from build123d import *

# Parameters (mm, degrees)
F1_DEPTH = 45
F2_W     = 30
F2_H     = 13
F3_DEPTH = 3
F4_W     = 2.1
F4_H     = 6
F5_DEPTH = 11
F7_D     = 2.83
F7_DEPTH = 2
F7_TIP   = 0.8502177759
F8_W     = 2
F8_H     = 45
F9_DEPTH = 1.5
F10_R    = 0.5


with BuildPart() as f1:
    # F0 (on Front) → F1 (new body)
    with BuildSketch(Plane.XZ):
        Polygon((0, 16), (0, 0), (20, 0), (20, 1.5), (3, 1.5), (1.5, 16), align=None)
    extrude(amount=F1_DEPTH)

    # F2 (on face) → F3 (join)
    with BuildSketch(Plane(origin=(0, 0, 0), x_dir=(0, -1, 0), z_dir=(-1, 0, 0))):
        with Locations((22.5, 6.5)):
            Rectangle(F2_W, F2_H)
    extrude(amount=F3_DEPTH)

    # F4 (on face) → F5 (cut)
    with BuildSketch(Plane(origin=(0, 0, 0), x_dir=(1, 0, 0), z_dir=(0, 0, -1))):
        with Locations((-1.05, 33.5)):
            Rectangle(F4_W, F4_H)
        with Locations((-1.05, 22.5)):
            Rectangle(F4_W, F4_H)
        with Locations((-1.05, 11.5)):
            Rectangle(F4_W, F4_H)
    extrude(amount=-F5_DEPTH, mode=Mode.SUBTRACT)

    # F7
    with Locations(Plane(origin=(-3, 0, 0), x_dir=(0, -1, 0), z_dir=(-1, 0, 0))):
        with Locations((33.5, 7), (22.5, 7), (11.5, 7)):
            Hole(F7_D / 2, depth=F7_DEPTH)
            with Locations((0, 0, -(F7_DEPTH + F7_TIP / 2))):  # 118° drill point
                Cone(0, F7_D / 2, F7_TIP, mode=Mode.SUBTRACT)

    # F8 (on face) → F9 (join)
    with BuildSketch(Plane.XY.offset(1.5)):
        with Locations((17.5, -22.5)):
            Rectangle(F8_W, F8_H)
    extrude(amount=F9_DEPTH)

    # F10
    f10_edges = [f1.edges().sort_by_distance(p)[0] for p in [
        (18.5, -22.5, 3),
        (16.5, -22.5, 3),
    ]]
    fillet(f10_edges, radius=F10_R)


solid = f1.part
The listing builds one solid part. Answer for the finished solid, in the listing's coordinates (mm). A direction names the side the tool comes from. Coordinates: 2 decimals unless noted, no trailing zeros. Write each loop counter-clockwise with the first axis right and the second up, starting at its lowest first coordinate (ties: lowest second). Pieces come first, ordered by that corner, then holes. Notation, with made-up numbers: M 57,71.25 L 100,71.25 A14 ccw 100,94.25 Z; hole C -17.75,-20 d10. An arc over 180 degrees is marked long. Put each result on its own line as item: value. Start each with the question number.
1. For a pull along X with two mould halves and no side action, classify faces 1 (the flat face through (-3, -22, 5)), 2 (the flat face through (0, -22, 5)), 3 (the flat face through (-1, -22, 13)), 4 (the flat face through (-1, -25.5, 5)) as pulls with the +X half, pulls with the -X half, needs draft (parallel to the pull), parting line crosses it, or undercut.
2. Flat-ended cylindrical pins translate along their axes: P1, Ø1, axis at x = -1, z = 5.5, coming from the -Y side; P2, Ø2, axis at y = -26.5, z = 8, coming from the +X side; P3, Ø6.5, axis at y = -23, z = 7, coming from the +X side. Find the tip coordinate at first contact, or state that the pin passes through.
3. A cutting plane is placed at C-C on x = 17.5. Write down the section's boundary in (y, z).
4. A cutting plane is placed at D-D on y = -27.5. Write down the section's boundary in (x, z), then the cut area to 3 significant figures.
5. A cutting plane is placed at A-A on y = -22.5. Write down the section's boundary in (x, z) (3 decimals), then the cut area to 3 significant figures.
6. A cutting plane is placed at B-B on z = 10. Write down the section's boundary in (x, y), then the cut area to 3 significant figures.
7. Which of the six approach directions +Z, -Z, +X, -X, +Y, -Y give full straight-line access (tool end or side, diameter ignored) to faces 5 (the flat face through (-1, -7.5, 6)), 6 (the cylindrical face through (-2.544, -34.623, 6.139)), 7 (the flat face through (10, -22, 1.5)), 8 (the flat face through (0, -17.2, 13.4)), 9 (the flat face through (-2.1, -22, 5))?
8. Consider line 1 (Z direction, x = -2.35, y = -22.5) (3 decimals); line 2 (Z direction, x = 14.5, y = -27); line 3 (X direction, y = -21.5, z = 10.5). Determine where each line is inside the solid, lowest interval first. Write a range as from..to.
Resolved:
1. face 1: pulls with the -X half
1. face 2: undercut
1. face 3: needs draft
1. face 4: undercut
2. P1: stops at y = -37.5
2. P2: stops at x = 2.43
2. P3: stops at x = 2.77
3. outline: M -45,0 L 0,0 L 0,3 L -45,3 Z
4. outline: M -3,0 L 20,0 L 20,1.5 L 18.5,1.5 L 18.5,2.5 A0.5 ccw 18,3 L 17,3 A0.5 ccw 16.5,2.5 L 16.5,1.5 L 3,1.5 L 1.5,16 L 0,16 L 0,13 L -3,13 Z
4. area: 105 mm2
5. outline: M -3,0 L -2.1,0 L -2.1,5.585 L -3,5.585 Z; M -3,8.415 L -2.1,8.415 L -2.1,11 L 0,11 L 0,0 L 20,0 L 20,1.5 L 18.5,1.5 L 18.5,2.5 A0.5 ccw 18,3 L 17,3 A0.5 ccw 16.5,2.5 L 16.5,1.5 L 3,1.5 L 1.5,16 L 0,16 L 0,13 L -3,13 Z
5. area: 78.9 mm2
6. outline: M -3,-37.5 L 0,-37.5 L 0,-45 L 2.12,-45 L 2.12,0 L 0,0 L 0,-7.5 L -3,-7.5 Z; hole M -2.1,-36.5 L 0,-36.5 L 0,-30.5 L -2.1,-30.5 Z; hole M -2.1,-25.5 L 0,-25.5 L 0,-19.5 L -2.1,-19.5 Z; hole M -2.1,-14.5 L 0,-14.5 L 0,-8.5 L -2.1,-8.5 Z
6. area: 148 mm2
7. face 5: +Z, -Z, -X, +Y
7. face 6: -X
7. face 7: +Z, +Y, -Y
7. face 8: +Z, -X
7. face 9: -Z
8. line 1: z = 0..5.585, 8.415..13
8. line 2: z = 0..1.5
8. line 3: x = -3..-2.1, 0..2.07
